The listing builds one solid part. Answer for the finished solid, in the listing's coordinates (mm). A direction names the side the tool comes from. Round coordinates to 2 decimals unless told otherwise and drop trailing zeros. Loops run counter-clockwise (first coordinate to the right, second up) from the corner with the lowest first, then second, coordinate; pieces in that order, holes last. Notation, with made-up numbers: (49.5, 26) -> (106.5, 26) arc R19 cw to (106.5, 39) -> close; hole circle Ø8 at (-35.75, 28.5). An arc over 180 degrees is marked (long way). Use a Markdown table: item, result. Add a question column.
Q1. Which of the six approach directions +Z, -Z, +X, -X, +Y, -Y give full straight-line access (tool end or side, diameter ignored) to faces 4 (the flat face through (145, 20, 28.5)), 5 (the flat face through (145, 20, 18.5)), 6 (the flat face through (51, 23, 32.5)), 7 (the flat face through (145, 20, -27.5)), 8 (the flat face through (145, 15, 24))?
Q2. Section B-B on z = -14.5 is taken. Give the vertices of the cut face in (x, y).
Q3. Section A-A on z = 0 is taken. Give the vertices of the cut face in (x, y), then the cut area to 3 significant figures.
Q4. For a pull along Z with two mould halves and no side action, classify faces 1 (the flat face through (150, 20, 24)), 2 (the flat face through (37, 9, -34.5)), 3 (the flat face through (39, 12, -37.5)) as released by +Z, released by -Z, zero draft, split by the parting line, or undercut.
Q5. Section D-D on z = -23.5 is taken. Give the vertices of the cut face in (x, y).
Q6. Given pin 1 Ø21.5 at (x, z) = (-44.5, -2) entering from -Y; pin 2 Ø14.5 at (y, z) = (5, 3.5) entering from -X; pin 3 Ø2 at (y, z) = (18.5, 21) entering from -X; pin 4 Ø8 at (x, y) = (142.5, 20.5) entering from -Z, each flat-ended and moving along its own axis, determine where each tip first touches the part or whether it passes through.
Q7. Section C-C on x = -45 is taken. Give the vertices of the cut face in (y, z).
Q8. Consider line 1 (X direction, y = 23.55, z = -14.5); line 2 (Z direction, x = 3.5, y = 5.5); line 3 (Z direction, x = 29.5, y = 23.25). Determine where each line is inside the solid, lowest interval first.
from build123d import *

# Parameters (mm, degrees)
SKETCH1_W           = 200
SKETCH1_H           = 75
BOSS_EXTRUDE1_DEPTH = 25
SKETCH9_W           = 165
SKETCH9_H           = 65
CUT_EXTRUDE5_DEPTH  = 4
SHELL3_START        = -34.5
SHELL3_DEPTH        = 69
SKETCH14_W          = 10
SKETCH14_H          = 10
BOSS_EXTRUDE5_DEPTH = 10
SKETCH15_R          = 5
CUT_EXTRUDE7_DEPTH  = 157.036053526
SKETCH16_W          = 20
SKETCH16_H          = 20
CUT_EXTRUDE8_DEPTH  = 157.624551077
SKETCH19_RX         = 5.75
SKETCH19_RY         = 5.5
SKETCH21_R          = 2.5
CUT_EXTRUDE9_DEPTH  = 157.624551117


# Read off the part's stored shape, not the designer's step: Shell3
with BuildPart() as part:
    # Sketch1 → Boss-Extrude1 (new body)
    with BuildSketch(Plane(origin=(0, 0, 0), x_dir=(1, 0, 0), z_dir=(0, 1, 0))):
        with Locations((40, 0)):
            Rectangle(SKETCH1_W, SKETCH1_H)
    extrude(amount=BOSS_EXTRUDE1_DEPTH)

    # Sketch9 → Cut-Extrude5 (cut)
    with BuildSketch(Plane(origin=(0, 25, 0), x_dir=(1, 0, 0), z_dir=(0, 1, 0))):
        with Locations((52.5, 0)):
            Rectangle(SKETCH9_W, SKETCH9_H)
    extrude(amount=-CUT_EXTRUDE5_DEPTH, mode=Mode.SUBTRACT)

    # Shell3 outline → Shell3 (cut)
    with BuildSketch(Plane.XY.offset(SHELL3_START)):
        Polygon((137, 0), (137, 18), (-33, 18), (-33, 22), (-60, 22), (-60, 0), align=None)
    extrude(amount=SHELL3_DEPTH, mode=Mode.SUBTRACT)

    # Sketch14 → Boss-Extrude5 (add)
    with BuildSketch(Plane(origin=(140, 0, 0), x_dir=(0, 0, -1), z_dir=(1, 0, 0))):
        with Locations((-23.5, 20)):
            Rectangle(SKETCH14_W, SKETCH14_H)
        with Locations((22.5, 20)):
            Rectangle(SKETCH14_W, SKETCH14_H)
    extrude(amount=BOSS_EXTRUDE5_DEPTH)

    # Sketch15 → Cut-Extrude7 (cut, through all)
    with BuildSketch(Plane(origin=(0, 21, 0), x_dir=(1, 0, 0), z_dir=(0, 1, 0))):
        with Locations(Location((-17.28231035, 0, 0), (0, 0, 270))):
            Circle(SKETCH15_R)
    extrude(amount=-CUT_EXTRUDE7_DEPTH, mode=Mode.SUBTRACT)

    # Sketch16 → Cut-Extrude8 (cut, through all)
    with BuildSketch(Plane(origin=(0, 25, 0), x_dir=(1, 0, 0), z_dir=(0, 1, 0))):
        with Locations((-45, 0)):
            Rectangle(SKETCH16_W, SKETCH16_H)
    extrude(amount=-CUT_EXTRUDE8_DEPTH, mode=Mode.SUBTRACT)

    # Cut-Sweep2: sweep along a path in Sketch20
    with BuildLine() as cut_sweep2_path:  # in the path sketch's own coordinates; laid on its plane below (add() does not lay a ready-made edge on the line's plane)
        add(Edge.make_bspline(
            [(-140, 6), (-136.19888528, 6.630281352), (-133.075750061, 4.182881523)],
            knots=[0, 0, 0, 1, 1, 1], degree=2))
    # Sketch19 → Cut-Sweep2 (sweep, cut)
    with BuildSketch(Plane(origin=(140, 0, 0), x_dir=(0, 0, -1), z_dir=(1, 0, 0))):
        with Locations(Location((-12.5, 6), (0, 0, 0))):
            Ellipse(SKETCH19_RX, SKETCH19_RY)
    sweep(path=Plane(origin=(0, 0, 0), x_dir=(-1, 0, 0), z_dir=(0, 0, -1)) * cut_sweep2_path.line, mode=Mode.SUBTRACT)

    # Sketch21 → Cut-Extrude9 (cut, through all)
    with BuildSketch(Plane(origin=(0, 25, 0), x_dir=(1, 0, 0), z_dir=(0, 1, 0))):
        with Locations(Location((-45, 14.5, 0), (0, 0, 270))):
            Circle(SKETCH21_R)
    extrude(amount=-CUT_EXTRUDE9_DEPTH, mode=Mode.SUBTRACT)


solid = part.part
Checked values:
| question | item | result |
|---|---|---|
| 1 | face 4 | +Z, +X, +Y, -Y |
| 1 | face 5 | +X, +Y, -Y |
| 1 | face 6 | +Y |
| 1 | face 7 | -Z, +X, +Y, -Y |
| 1 | face 8 | +Z, -Z, +X, -Y |
| 2 | outline | (-60, 22) -> (-47.5, 22) -> (-47.5, 25) -> (-60, 25) -> close; (-42.5, 22) -> (-33, 22) -> (-33, 18) -> (137, 18) -> (137, 0) -> (140, 0) -> (140, 25) -> (135, 25) -> (135, 21) -> (-30, 21) -> (-30, 25) -> (-42.5, 25) -> close |
| 3 | outline | (-60, 22) -> (-55, 22) -> (-55, 25) -> (-60, 25) -> close; (-35, 22) -> (-33, 22) -> (-33, 18) -> (-22.28, 18) -> (-22.28, 21) -> (-30, 21) -> (-30, 25) -> (-35, 25) -> close; (-12.28, 18) -> (137, 18) -> (137, 0) -> (140, 0) -> (140, 25) -> (135, 25) -> (135, 21) -> (-12.28, 21) -> close |
| 3 | area | 596 mm2 |
| 4 | face 1 | zero draft |
| 4 | face 2 | undercut |
| 4 | face 3 | released by -Z |
| 5 | outline | (-60, 22) -> (-33, 22) -> (-33, 18) -> (137, 18) -> (137, 0) -> (140, 0) -> (140, 15) -> (150, 15) -> (150, 25) -> (135, 25) -> (135, 21) -> (-30, 21) -> (-30, 25) -> (-60, 25) -> close |
| 6 | pin 1 | stops at y = 22 |
| 6 | pin 2 | stops at x = 137 |
| 6 | pin 3 | stops at x = -33 |
| 6 | pin 4 | stops at z = -37.5 |
| 7 | outline | (0, -37.5) -> (25, -37.5) -> (25, -17) -> (22, -17) -> (22, -34.5) -> (0, -34.5) -> close; (0, 34.5) -> (22, 34.5) -> (22, 10) -> (25, 10) -> (25, 37.5) -> (0, 37.5) -> close; (22, -12) -> (25, -12) -> (25, -10) -> (22, -10) -> close |
| 8 | line 1 | x = -60 to -47.5, -42.5 to -30, 135 to 140 |
| 8 | line 2 | z = -37.5 to -34.5, 34.5 to 37.5 |
| 8 | line 3 | z = -37.5 to -32.5, 32.5 to 37.5 |
